Read the model definition and answer for the solid it produces. Units are mm, in the model's axes. Face numbers are marked on the shaded views. A direction names the side the tool comes from. Round coordinates to 2 decimals unless told otherwise and drop trailing zeros. Loops run counter-clockwise (first coordinate to the right, second up) from the corner with the lowest first, then second, coordinate; pieces in that order, holes last. Notation, with made-up numbers: M -22,67.25 L -12,67.25 A21 cw -12,98.25 Z; hole C -9.5,30 d8. An arc over 180 degrees is marked long. Answer as CSV lines item,"result".
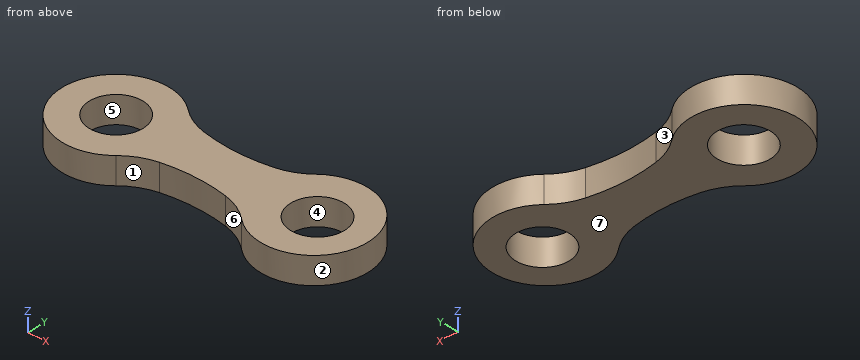
```python
from build123d import *

# Parameters (mm, degrees)
BOSS_EXTRUDE1_DEPTH = 3
SKETCH2_R           = 3
CUT_EXTRUDE1_DEPTH  = 3


with BuildPart() as part:
    # Sketch1 → Boss-Extrude1 (new body)
    with BuildSketch(Plane.XY):
        with BuildLine():
            ThreePointArc((-38.993072638, 10.297497813), (-29.003536718, 14.749442663), (-38.948867239, 19.299282405))
            ThreePointArc((-38.948867239, 19.299282405), (-40.43645285, 18.304531068), (-42.127647344, 17.719464956))
            ThreePointArc((-42.127647344, 17.719464956), (-46.049056408, 17.312851184), (-49.971869959, 17.705684038))
            ThreePointArc((-49.971869959, 17.705684038), (-51.638902703, 18.27196215), (-53.111913064, 19.236280328))
            ThreePointArc((-53.111913064, 19.236280328), (-63.002628538, 14.569315621), (-52.961652305, 10.235078841))
            ThreePointArc((-52.961652305, 10.235078841), (-51.409870812, 11.305926496), (-49.628578883, 11.923777258))
            ThreePointArc((-49.628578883, 11.923777258), (-45.958785243, 12.292784959), (-42.287798819, 11.935838578))
            ThreePointArc((-42.287798819, 11.935838578), (-40.530859131, 11.337028267), (-38.993072638, 10.297497813))
        make_face()
    extrude(amount=BOSS_EXTRUDE1_DEPTH)

    # Sketch2 → Cut-Extrude1 (cut)
    with BuildSketch(Plane.XY.offset(3)):
        with Locations((-57.001914988, 14.704587642)):
            Circle(SKETCH2_R)
        with Locations((-34.595484072, 14.749442663)):
            Circle(SKETCH2_R)
    extrude(amount=-CUT_EXTRUDE1_DEPTH, mode=Mode.SUBTRACT)


solid = part.part
```
1) Each of these flat-tipped pins is pushed along its axis until it touches: P1, Ø1, axis at x = -33, z = 0.5, coming from the -Y side; P2, Ø3.5, axis at x = -57, y = 14.7, coming from the +Z side; P3, Ø1.5, axis at y = 16.5, z = 2, coming from the -X side. Where does it stop, or does it pass through?
Evaluation:
P1,"stops at y = 8.97"
P2,"passes through"
P3,"stops at x = -62.91"
2) A tool of negligible diameter and unlimited length cuts with its end or side. For the marked faces 1, 2 and 3, from which of +Z, -Z, +X, -X, +Y, -Y can it reach the whole face along a straight path? Write none if from no direction.
Evaluation:
face 1,"+Z, -Z, -Y"
face 2,"+Z, -Z"
face 3,"+Z, -Z, +Y"
3) Find section C-C, the plane z = 0.95. Give the vertices of the cut face in (x, y), then the cut area to 3 significant figures.
Evaluation:
outline,"M -53.11,19.24 A6 ccw long -52.96,10.24 A7 cw -49.63,11.92 A18.74 cw -42.29,11.94 A7 cw -38.99,10.3 A6 ccw long -38.95,19.3 A7 cw -42.13,17.72 A19.44 cw -49.97,17.71 A7 cw Z; hole C -57,14.7 d6; hole C -34.6,14.75 d6"
area,"230 mm^2"
4) Straight lines are drawn through the part: line 1 (X direction, y = 14, z = 2.85); line 2 (X direction, y = 12.5, z = 0.45); line 3 (Y direction, x = -33, z = 0.7). For each, find the intervals that lie inside material, in ascending order.
Evaluation:
line 1,"x = -62.97 to -59.92, -54.09 to -37.5, -31.69 to -29.05"
line 2,"x = -62.6 to -59.04, -54.97 to -36.58, -32.61 to -29.45"
line 3,"y = 9.12 to 12.21, 17.29 to 20.43"
5) Find section A-A, the plane y = 20. Give the vertices of the cut face in (x, z).
Evaluation:
outline,"M -59.76,0 L -54.25,0 L -54.25,3 L -59.76,3 Z; M -37.96,0 L -32.05,0 L -32.05,3 L -37.96,3 Z"
6) Find section B-B, the plane x = -58. Give the vertices of the cut face in (y, z), then the cut area to 3 significant figures.
Evaluation:
outline,"M 8.75,0 L 11.88,0 L 11.88,3 L 8.75,3 Z; M 17.53,0 L 20.59,0 L 20.59,3 L 17.53,3 Z"
area,"18.5 mm^2"
7) Determine the mould class of the marked faces 4, 5, 6 and 7 for opening direction Y: released by +Y, released by -Y, zero draft, split by the parting line, or undercut.
Evaluation:
face 4,"undercut"
face 5,"undercut"
face 6,"released by -Y"
face 7,"zero draft"
8) Find section D-D, the plane x = -44. Give the vertices of the cut face in (y, z), then the cut area to 3 significant figures.
Evaluation:
outline,"M 12.19,0 L 17.42,0 L 17.42,3 L 12.19,3 Z"
area,"15.7 mm^2"
